Verification items for the finished model (mm, model axes). A direction names the side the tool comes from. Give positions to 0.01 mm unless a question says otherwise; leave off trailing zeros. Write each loop counter-clockwise with the first axis right and the second up, starting at its lowest first coordinate (ties: lowest second). Pieces come first, ordered by that corner, then holes. Notation, with made-up numbers: (-32.5, -12.75) -> (-1.5, -12.75) arc R25 ccw to (-1.5, 14.25) -> close; hole circle Ø10 at (69, 28). An arc over 180 degrees is marked (long way). Answer as CSV lines item,"result". Start each with the question number.
1) Tool access check on faces 4 (the flat face through (21.59, -13, 0)), 5 (the flat face through (-25.4, -5, 0)), 6 (the flat face through (7.62, -13, -14)), 7 (the flat face through (5.842, -13, 13)), 8 (the flat face through (25.4, -9, 0)). Record the directions out of +Z, -Z, +X, -X, +Y, -Y that give a thin tool (end or side, any length) a straight path to the whole face; none if there is none.
2) Gauge pin test, flat ends, axial feed: pin 1 Ø4 at (y, z) = (-13, -14.5) entering from +X; pin 2 Ø1.5 at (x, z) = (-18.5, -1) entering from -Y (3 decimals); pin 3 Ø12 at (y, z) = (-16, -15) entering from -X (3 decimals). Record the tip position at first contact, or that the pin passes through.
3) Sectioned sample at C-C on x = 14. Record the cut outline in (y, z).
4) Material ranges on L1, parallel to X at y = 4.5, z = 12.7; L2, parallel to X at y = -10.25, z = -6.5 (3 decimals); L3, parallel to X at y = -16.5, z = 0 (3 decimals), recorded low to high.
5) Sectioned sample at D-D on y = 3.5. Record the cut outline in (x, z), and give its area (3 significant figures).
6) Sectioned sample at B-B on z = -12.7. Record the cut outline in (x, y) (3 decimals), and give its area (3 significant figures).
7) Sectioned sample at A-A on y = -14. Record the cut outline in (x, z) (3 decimals), and give its area (3 significant figures).
8) Mould release check, pull along Z, two halves, no side actions. Record for faces 1 (the cylindrical face through (33.13, 3.22, -12.98)), 2 (the flat face through (-1, -4, 19.05)), 3 (the flat face through (6, -19.05, 0)): released by +Z, released by -Z, zero draft, split by the parting line, or undercut.
```python
from build123d import *

# Parameters (mm, degrees)
SKETCH1_W           = 88.9
SKETCH1_H           = 38.1
BOSS_EXTRUDE1_DEPTH = 6.35
CUT_EXTRUDE1_REACH  = 50.775
SKETCH2_R           = 2.159
SKETCH3_W           = 50.8
SKETCH3_H           = 38.1
BOSS_EXTRUDE2_DEPTH = 19.05
SKETCH4_W           = 22.225
SKETCH4_H           = 38.1
CUT_EXTRUDE2_DEPTH  = 9.525
CUT_EXTRUDE3_DEPTH  = 12.7


with BuildPart() as part:
    # Sketch1 → Boss-Extrude1 (new body)
    with BuildSketch(Plane(origin=(0, 0, 0), x_dir=(1, 0, 0), z_dir=(0, 1, 0))):
        Rectangle(SKETCH1_W, SKETCH1_H)
    extrude(amount=BOSS_EXTRUDE1_DEPTH)

    # Sketch2 → Cut-Extrude1 (cut, up to next)
    with BuildSketch(Plane(origin=(0, 6.35, 0), x_dir=(1, 0, 0), z_dir=(0, 1, 0)), mode=Mode.PRIVATE) as cut_extrude1_sk1:
        with Locations(Location((-30.988, 12.7, 0), (0, 0, 270))):
            Circle(SKETCH2_R)
    cut_extrude1_tool1 = extrude(cut_extrude1_sk1.sketch, amount=-CUT_EXTRUDE1_REACH, mode=Mode.PRIVATE) & part.part
    # Sketch2 → Cut-Extrude1 (cut, up to next)
    with BuildSketch(Plane(origin=(0, 6.35, 0), x_dir=(1, 0, 0), z_dir=(0, 1, 0)), mode=Mode.PRIVATE) as cut_extrude1_sk2:
        with Locations(Location((30.988, 12.7, 0), (0, 0, 270))):
            Circle(SKETCH2_R)
    cut_extrude1_tool2 = extrude(cut_extrude1_sk2.sketch, amount=-CUT_EXTRUDE1_REACH, mode=Mode.PRIVATE) & part.part
    # Sketch2 → Cut-Extrude1 (cut, up to next)
    with BuildSketch(Plane(origin=(0, 6.35, 0), x_dir=(1, 0, 0), z_dir=(0, 1, 0)), mode=Mode.PRIVATE) as cut_extrude1_sk3:
        with Locations(Location((30.988, -12.7, 0), (0, 0, 270))):
            Circle(SKETCH2_R)
    cut_extrude1_tool3 = extrude(cut_extrude1_sk3.sketch, amount=-CUT_EXTRUDE1_REACH, mode=Mode.PRIVATE) & part.part
    # Sketch2 → Cut-Extrude1 (cut, up to next)
    with BuildSketch(Plane(origin=(0, 6.35, 0), x_dir=(1, 0, 0), z_dir=(0, 1, 0)), mode=Mode.PRIVATE) as cut_extrude1_sk4:
        with Locations(Location((-30.988, -12.7, 0), (0, 0, 270))):
            Circle(SKETCH2_R)
    cut_extrude1_tool4 = extrude(cut_extrude1_sk4.sketch, amount=-CUT_EXTRUDE1_REACH, mode=Mode.PRIVATE) & part.part
    add(cut_extrude1_tool1.solids().sort_by_distance((-30.988, 6.35, -12.7))[0], mode=Mode.SUBTRACT)
    add(cut_extrude1_tool2.solids().sort_by_distance((30.988, 6.35, -12.7))[0], mode=Mode.SUBTRACT)
    add(cut_extrude1_tool3.solids().sort_by_distance((30.988, 6.35, 12.7))[0], mode=Mode.SUBTRACT)
    add(cut_extrude1_tool4.solids().sort_by_distance((-30.988, 6.35, 12.7))[0], mode=Mode.SUBTRACT)

    # Sketch3 → Boss-Extrude2 (add)
    with BuildSketch(Plane.XZ):
        Rectangle(SKETCH3_W, SKETCH3_H)
    extrude(amount=BOSS_EXTRUDE2_DEPTH)

    # Sketch4 → Cut-Extrude2 (cut)
    with BuildSketch(Plane(origin=(0, -19.05, 0), x_dir=(-1, 0, 0), z_dir=(0, -1, 0))):
        with Locations((14.2875, 0)):
            Rectangle(SKETCH4_W, SKETCH4_H)
    extrude(amount=-CUT_EXTRUDE2_DEPTH, mode=Mode.SUBTRACT)

    # Sketch5 → Cut-Extrude3 (cut)
    with BuildSketch(Plane.XZ.offset(19.05)):
        Polygon((5.842, -19.05), (5.842, -6.35), (19.812, -6.35), (19.812, 6.35), (5.842, 6.35), (5.842, 19.05), (7.62, 19.05), (7.62, 8.128), (21.59, 8.128), (21.59, -8.128), (7.62, -8.128), (7.62, -19.05), align=None)
    extrude(amount=-CUT_EXTRUDE3_DEPTH, mode=Mode.SUBTRACT)


solid = part.part
```
Ans:
1,face 4,"-Y"
1,face 5,"+Z, -Z, -X, -Y"
1,face 6,"-Z, -Y"
1,face 7,"+Z, -Y"
1,face 8,"+Z, -Z, +X, -Y"
2,pin 1,"stops at x = 25.4"
2,pin 2,"stops at y = -9.525"
2,pin 3,"stops at x = -3.175"
3,outline,"(-19.05, -19.05) -> (6.35, -19.05) -> (6.35, 19.05) -> (-19.05, 19.05) -> (-19.05, 8.13) -> (-6.35, 8.13) -> (-6.35, 6.35) -> (-19.05, 6.35) -> (-19.05, -6.35) -> (-6.35, -6.35) -> (-6.35, -8.13) -> (-19.05, -8.13) -> close"
4,L1,"x = -44.45 to -33.15, -28.83 to 28.83, 33.15 to 44.45"
4,L2,"x = -3.175 to 5.842, 21.59 to 25.4"
4,L3,"x = -3.175 to 19.812, 21.59 to 25.4"
5,outline,"(-44.45, -19.05) -> (44.45, -19.05) -> (44.45, 19.05) -> (-44.45, 19.05) -> close; hole circle Ø4.32 at (-30.99, -12.7); hole circle Ø4.32 at (-30.99, 12.7); hole circle Ø4.32 at (30.99, -12.7); hole circle Ø4.32 at (30.99, 12.7)"
5,area,"3,330 mm²"
6,outline,"(-44.45, 0) -> (-33.147, 0) -> (-33.147, 6.35) -> (-44.45, 6.35) -> close; (-28.829, 0) -> (-25.4, 0) -> (-25.4, -9.525) -> (-3.175, -9.525) -> (-3.175, -19.05) -> (5.842, -19.05) -> (5.842, -6.35) -> (7.62, -6.35) -> (7.62, -19.05) -> (25.4, -19.05) -> (25.4, 0) -> (28.829, 0) -> (28.829, 6.35) -> (-28.829, 6.35) -> close; (33.147, 0) -> (44.45, 0) -> (44.45, 6.35) -> (33.147, 6.35) -> close"
6,area,"1,240 mm²"
7,outline,"(-3.175, -19.05) -> (5.842, -19.05) -> (5.842, -6.35) -> (19.812, -6.35) -> (19.812, 6.35) -> (5.842, 6.35) -> (5.842, 19.05) -> (-3.175, 19.05) -> close; (7.62, -19.05) -> (25.4, -19.05) -> (25.4, 19.05) -> (7.62, 19.05) -> (7.62, 8.128) -> (21.59, 8.128) -> (21.59, -8.128) -> (7.62, -8.128) -> close"
7,area,"971 mm²"
8,face 1,"undercut"
8,face 2,"released by +Z"
8,face 3,"zero draft"
